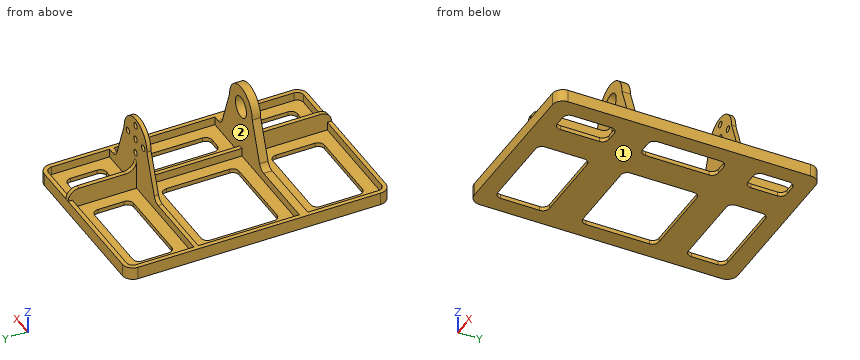
```python
from build123d import *

# Parameters (mm, degrees)
PAD_DEPTH    = 2
SKETCH001_R  = 5.1
PAD001_DEPTH = 4
SKETCH002_R  = 1.5
PAD002_DEPTH = 2
SKETCH003_W  = 4
SKETCH003_H  = 48
PAD003_DEPTH = 1
PAD004_DEPTH = 4


with BuildPart() as part:
    # Sketch → Pad (new body)
    with BuildSketch(Plane.XY):
        with BuildLine():
            ThreePointArc((-36, 62.5), (-39.535534, 61.035534), (-41, 57.5))
            Line((-41, -57.5), (-41, 57.5))
            ThreePointArc((-41, -57.5), (-39.535534, -61.035534), (-36, -62.5))
            Line((36, -62.5), (-36, -62.5))
            ThreePointArc((36, -62.5), (39.535534, -61.035534), (41, -57.5))
            Line((41, 57.5), (41, -57.5))
            ThreePointArc((41, 57.5), (39.535534, 61.035534), (36, 62.5))
            Line((-36, 62.5), (36, 62.5))
        make_face()
        with BuildLine():
            ThreePointArc((-30, 54.5), (-32.12132, 53.62132), (-33, 51.5))
            Line((-33, 39), (-33, 51.5))
            ThreePointArc((-33, 39), (-32.12132, 36.87868), (-30, 36))
            Line((5, 36), (-30, 36))
            ThreePointArc((5, 36), (7.12132, 36.87868), (8, 39))
            Line((8, 51.5), (8, 39))
            ThreePointArc((8, 51.5), (7.12132, 53.62132), (5, 54.5))
            Line((-30, 54.5), (5, 54.5))
        make_face(mode=Mode.SUBTRACT)
        with BuildLine():
            ThreePointArc((25, 54.5), (22.87868, 53.62132), (22, 51.5))
            Line((22, 39), (22, 51.5))
            ThreePointArc((22, 39), (22.87868, 36.87868), (25, 36))
            Line((30, 36), (25, 36))
            ThreePointArc((30, 36), (32.12132, 36.87868), (33, 39))
            Line((33, 51.5), (33, 39))
            ThreePointArc((33, 51.5), (32.12132, 53.62132), (30, 54.5))
            Line((25, 54.5), (30, 54.5))
        make_face(mode=Mode.SUBTRACT)
        with BuildLine():
            ThreePointArc((-30, 22), (-32.12132, 21.12132), (-33, 19))
            Line((-33, -11), (-33, 19))
            ThreePointArc((-33, -11), (-32.12132, -13.12132), (-30, -14))
            Line((5, -14), (-30, -14))
            ThreePointArc((5, -14), (7.12132, -13.12132), (8, -11))
            Line((8, 19), (8, -11))
            ThreePointArc((8, 19), (7.12132, 21.12132), (5, 22))
            Line((-30, 22), (5, 22))
        make_face(mode=Mode.SUBTRACT)
        with BuildLine():
            ThreePointArc((25, 22), (22.87868, 21.12132), (22, 19))
            Line((22, -11), (22, 19))
            ThreePointArc((22, -11), (22.87868, -13.12132), (25, -14))
            Line((30, -14), (25, -14))
            ThreePointArc((30, -14), (32.12132, -13.12132), (33, -11))
            Line((33, 19), (33, -11))
            ThreePointArc((33, 19), (32.12132, 21.12132), (30, 22))
            Line((25, 22), (30, 22))
        make_face(mode=Mode.SUBTRACT)
        with BuildLine():
            ThreePointArc((-30, -30), (-32.12132, -30.87868), (-33, -33))
            Line((-33, -51.5), (-33, -33))
            ThreePointArc((-33, -51.5), (-32.12132, -53.62132), (-30, -54.5))
            Line((5, -54.5), (-30, -54.5))
            ThreePointArc((5, -54.5), (7.12132, -53.62132), (8, -51.5))
            Line((8, -33), (8, -51.5))
            ThreePointArc((8, -33), (7.12132, -30.87868), (5, -30))
            Line((-30, -30), (5, -30))
        make_face(mode=Mode.SUBTRACT)
        with BuildLine():
            ThreePointArc((25, -30), (22.87868, -30.87868), (22, -33))
            Line((22, -51.5), (22, -33))
            ThreePointArc((22, -51.5), (22.87868, -53.62132), (25, -54.5))
            Line((30, -54.5), (25, -54.5))
            ThreePointArc((30, -54.5), (32.12132, -53.62132), (33, -51.5))
            Line((33, -33), (33, -51.5))
            ThreePointArc((33, -33), (32.12132, -30.87868), (30, -30))
            Line((25, -30), (30, -30))
        make_face(mode=Mode.SUBTRACT)
    extrude(amount=PAD_DEPTH)

    # Sketch001 (on DatumPlane) → Pad001 (join)
    with BuildSketch(Plane.XZ.offset(24)):
        with BuildLine():
            Line((39, 2), (39, 6))
            Line((39, 6), (36, 6))
            ThreePointArc((32.244908, 8.621855), (33.710085, 6.720322), (36, 6))
            Line((32.244908, 8.621855), (25.5, 27))
            ThreePointArc((25.5, 27), (15, 37.5), (4.5, 27))
            Line((4.5, 27), (-2.244908, 8.621855))
            ThreePointArc((-6, 6), (-3.710085, 6.720322), (-2.244908, 8.621855))
            Line((-6, 6), (-39, 6))
            Line((-39, 6), (-39, 2))
            Line((-39, 2), (39, 2))
        make_face()
        with Locations((15, 27)):
            Circle(SKETCH001_R, mode=Mode.SUBTRACT)
    extrude(amount=-PAD001_DEPTH)

    # Sketch002 (on DatumPlane) → Pad002 (join)
    with BuildSketch(Plane.XZ.offset(-28)):
        with BuildLine():
            Line((-39, 2), (39, 2))
            Line((39, 2), (39, 6))
            Line((36, 6), (39, 6))
            ThreePointArc((32.244908, 8.621855), (33.710085, 6.720322), (36, 6))
            Line((25.5, 27), (32.244908, 8.621855))
            ThreePointArc((25.5, 27), (15, 37.5), (4.5, 27))
            Line((-2.244908, 8.621855), (4.5, 27))
            ThreePointArc((-6, 6), (-3.710085, 6.720322), (-2.244908, 8.621855))
            Line((-39, 6), (-6, 6))
            Line((-39, 2), (-39, 6))
        make_face()
        with Locations((7.928932, 27)):
            Circle(SKETCH002_R, mode=Mode.SUBTRACT)
        with Locations((15, 34.071068)):
            Circle(SKETCH002_R, mode=Mode.SUBTRACT)
        with Locations((15, 27)):
            Circle(SKETCH002_R, mode=Mode.SUBTRACT)
        with Locations((22.071068, 27)):
            Circle(SKETCH002_R, mode=Mode.SUBTRACT)
        with Locations((15, 19.928932)):
            Circle(SKETCH002_R, mode=Mode.SUBTRACT)
    extrude(amount=-PAD002_DEPTH)

    # Sketch003 (on DatumPlane) → Pad003 (join, symmetric)
    with BuildSketch(Plane(origin=(15, -24, 26), x_dir=(0, 0, 1), z_dir=(1, 0, 0))):
        with BuildLine():
            Line((-24, -54), (-24, -86.5))
            Line((-24, -86.5), (-20, -86.5))
            ThreePointArc((-20, -86.5), (-16.312816, -84.972718), (-14.785534, -81.285534))
            Line((-14.785534, -59.214466), (-14.785534, -81.285534))
            ThreePointArc((-9.571068, -54), (-13.258252, -55.527282), (-14.785534, -59.214466))
            Line((-24, -54), (-9.571068, -54))
        make_face()
        with BuildLine():
            Line((-24, 38.5), (-24, 0))
            Line((-24, 0), (-9.571068, 0))
            ThreePointArc((-14.785534, 5.214466), (-13.258252, 1.527282), (-9.571068, 0))
            Line((-14.785534, 33.285534), (-14.785534, 5.214466))
            ThreePointArc((-14.785534, 33.285534), (-16.312816, 36.972718), (-20, 38.5))
            Line((-24, 38.5), (-20, 38.5))
        make_face()
        with Locations((-22, -28)):
            Rectangle(SKETCH003_W, SKETCH003_H)
    extrude(amount=PAD003_DEPTH, both=True)

    # Sketch004 (on Face8 of Pad003) → Pad004 (join)
    with BuildSketch(Plane.XY.offset(2)):
        with BuildLine():
            Line((-41, -57.5), (-41, 57.5))
            ThreePointArc((-36, 62.5), (-39.535534, 61.035534), (-41, 57.5))
            Line((-36, 62.5), (14, 62.5))
            Line((14, 60.5), (14, 62.5))
            Line((14, 60.5), (-36, 60.5))
            ThreePointArc((-36, 60.5), (-38.12132, 59.62132), (-39, 57.5))
            Line((-39, 57.5), (-39, -57.5))
            ThreePointArc((-39, -57.5), (-38.12132, -59.62132), (-36, -60.5))
            Line((14, -60.5), (-36, -60.5))
            Line((14, -62.5), (14, -60.5))
            Line((-36, -62.5), (14, -62.5))
            ThreePointArc((-41, -57.5), (-39.535534, -61.035534), (-36, -62.5))
        make_face()
        with BuildLine():
            Line((16, 62.5), (36, 62.5))
            ThreePointArc((41, 57.5), (39.535534, 61.035534), (36, 62.5))
            Line((41, -57.5), (41, 57.5))
            ThreePointArc((36, -62.5), (39.535534, -61.035534), (41, -57.5))
            Line((16, -62.5), (36, -62.5))
            Line((16, -60.5), (16, -62.5))
            Line((16, -60.5), (36, -60.5))
            ThreePointArc((36, -60.5), (38.12132, -59.62132), (39, -57.5))
            Line((39, 57.5), (39, -57.5))
            ThreePointArc((39, 57.5), (38.12132, 59.62132), (36, 60.5))
            Line((36, 60.5), (16, 60.5))
            Line((16, 60.5), (16, 62.5))
        make_face()
    extrude(amount=PAD004_DEPTH)


solid = part.part
```
Could you check a few things on this model? Use its own coordinates, in mm. Face numbers are marked on the shaded views. Round coordinates to 2 decimals unless told otherwise and drop trailing zeros. Write each loop counter-clockwise with the first axis right and the second up, starting at its lowest first coordinate (ties: lowest second). Pieces come first, ordered by that corner, then holes. Notation, with made-up numbers: M -17.75,33 L 37.25,33 A30 ccw 37.25,64 Z; hole C 75.5,83.5 d2. An arc over 180 degrees is marked long. Answer in a Markdown table with one row per item. Add a question column.
Q1. Imagine slicing it at C-C (y = -17.5). Please give me the cut outline in (x, z), then the cut area to 3 significant figures.
Q2. If we mould it in two halves opening along X, with no side actions, what happens to the marked faces 1 and 2? For each: +X half, -X half, draft (parallel to the pull), parting line (faces both ways), or undercut.
Q3. Imagine slicing it at B-B (x = -13). Please give me the cut outline in (y, z), then the cut area to 3 significant figures.
Q4. If I drill on line 1 (Y direction, x = 5, z = 5); line 2 (X direction, y = 24, z = 3); line 3 (Z direction, x = 15, y = 28.75), over which ranges is the centre line in solid material (lowest first)? Write a range as from..to.
Q5. Imagine slicing it at A-A (y = 4). Please give me the cut outline in (x, z).
Q6. Imagine slicing it at D-D (x = 2.5). Please give me the cut outline in (y, z).
Q7. Will these pins go through, and if not, where does the flat tip stop? pin 1 Ø7.5 at (x, y) = (26, -6.5) entering from +Z; pin 2 Ø5 at (x, z) = (15, 34.07) entering from -Y; pin 3 Ø11.5 at (y, z) = (-37.5, 11.5) entering from +X; pin 4 Ø24 at (x, y) = (-6, -6.5) entering from +Z.
Values:
| question | item | result |
|---|---|---|
| 1 | outline | M -41,0 L 41,0 L 41,6 L 39,6 L 39,2 L 16,2 L 16,6 L 14,6 L 14,2 L -39,2 L -39,6 L -41,6 Z |
| 1 | area | 188 mm^2 |
| 2 | face 1 | draft |
| 2 | face 2 | undercut |
| 3 | outline | M -62.5,0 L -54.5,0 L -54.5,2 L -60.5,2 L -60.5,6 L -62.5,6 Z; M -30,0 L -14,0 L -14,2 L -20,2 L -20,6 L -24,6 L -24,2 L -30,2 Z; M 22,0 L 36,0 L 36,2 L 30,2 L 30,6 L 28,6 L 28,2 L 22,2 Z; M 54.5,0 L 62.5,0 L 62.5,6 L 60.5,6 L 60.5,2 L 54.5,2 Z |
| 3 | area | 132 mm^2 |
| 4 | line 1 | -62.5..-60.5, -24..-20, 28..30, 60.5..62.5 |
| 4 | line 2 | -41..-39, 14..16, 39..41 |
| 4 | line 3 | 0..18.43, 21.43..25.5, 28.5..32.57, 35.57..37.5 |
| 5 | outline | M -41,0 L -33,0 L -33,2 L -39,2 L -39,6 L -41,6 Z; M 8,0 L 22,0 L 22,2 L 16,2 L 16,6 L 14,6 L 14,2 L 8,2 Z; M 33,0 L 41,0 L 41,6 L 39,6 L 39,2 L 33,2 Z |
| 6 | outline | M -62.5,0 L -54.5,0 L -54.5,2 L -60.5,2 L -60.5,6 L -62.5,6 Z; M -30,0 L -14,0 L -14,2 L -20,2 L -20,21.55 L -24,21.55 L -24,2 L -30,2 Z; M 22,0 L 36,0 L 36,2 L 30,2 L 30,21.55 L 28,21.55 L 28,2 L 22,2 Z; M 54.5,0 L 62.5,0 L 62.5,6 L 60.5,6 L 60.5,2 L 54.5,2 Z |
| 7 | pin 1 | through |
| 7 | pin 2 | y = -24 |
| 7 | pin 3 | x = 41 |
| 7 | pin 4 | z = 2 |
